Part model, mm, in its own coordinate system. Face numbers are marked on the shaded views. A direction names the side the tool comes from. Give positions to 0.01 mm unless a question says otherwise; leave off trailing zeros. Loops run counter-clockwise (first coordinate to the right, second up) from the corner with the lowest first, then second, coordinate; pieces in that order, holes last. Notation, with made-up numbers: M 79.25,70 L 83.25,70 A30 cw 83.25,105 Z; hole C -18,17.5 d4. An arc over 180 degrees is marked long. Answer in a Markdown table with one row per item.
from build123d import *

# Parameters (mm, degrees)
F0_W     = 40
F0_H     = 5
F1_DEPTH = 50
F0_W_2   = 30
F0_H_2   = 30
F2_DEPTH = 5


with BuildPart() as f1:
    # F0 (on Top) → F1 (new body)
    with BuildSketch(Plane.XY):
        Polygon((25, 10), (-25, 10), (-25, 0), (-15, 0), (15, 0), (25, 0), align=None)
        with Locations((0, 5)):
            Rectangle(F0_W, F0_H, mode=Mode.SUBTRACT)
    extrude(amount=F1_DEPTH)

    # F0 (on Top) → F2 (join)
    with BuildSketch(Plane.XY):
        with Locations((0, -15)):
            Rectangle(F0_W_2, F0_H_2)
        with Locations((0, 5)):
            Rectangle(F0_W, F0_H)
    extrude(amount=F2_DEPTH)


solid = f1.part
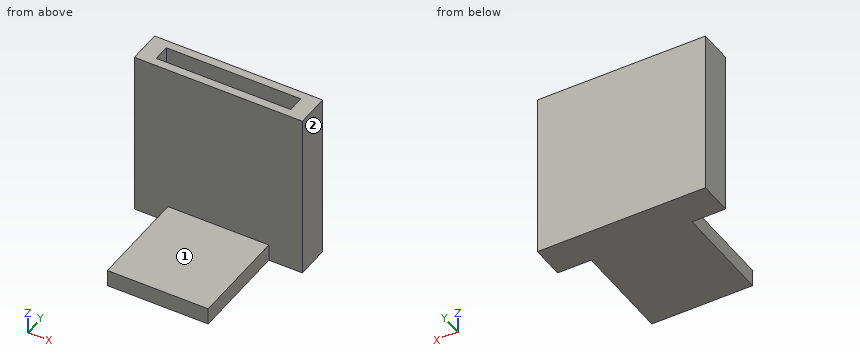
(1) Saw through at B-B (x = -16.5). Write the cut outline in (y, z), plus the area to 3 significant figures.
Recorded:
| item | result |
|---|---|
| outline | M 0,0 L 10,0 L 10,50 L 7.5,50 L 7.5,5 L 2.5,5 L 2.5,50 L 0,50 Z |
| area | 275 mm^2 |
(2) Saw through at C-C (y = 3.5). Write the cut outline in (x, z).
Recorded:
| item | result |
|---|---|
| outline | M -25,0 L 25,0 L 25,50 L 20,50 L 20,5 L -20,5 L -20,50 L -25,50 Z |
(3) Which spindle directions (+Z, -Z, +X, -X, +Y, -Y) get a long thin tool onto all of the face, cutting with end or side? Do the marked faces 1 and 2. Say none if no direction does.
Recorded:
| item | result |
|---|---|
| face 1 | +Z, +X, -X, -Y |
| face 2 | +Z, -Z, +X, +Y, -Y |
(4) Saw through at A-A (z = 8). Write the cut outline in (x, y), plus the area to 3 significant figures.
Recorded:
| item | result |
|---|---|
| outline | M -25,0 L 25,0 L 25,10 L -25,10 Z; hole M -20,2.5 L 20,2.5 L 20,7.5 L -20,7.5 Z |
| area | 300 mm^2 |
(5) Drill centre lines: line 1 along X through (y, z) = (7, 45); line 2 along Y through (x, z) = (-10, 11.5); line 3 along Z through (x, y) = (-1, -3). Where is each one in solid material? Low to high.
Recorded:
| item | result |
|---|---|
| line 1 | x = -25 to -20, 20 to 25 |
| line 2 | y = 0 to 2.5, 7.5 to 10 |
| line 3 | z = 0 to 5 |
(6) Pin check, flat tips, straight feed: pin 1 Ø2.5 at (y, z) = (-22, 3.5) entering from -X; pin 2 Ø1 at (x, z) = (15, 42.5) entering from -Y; pin 3 Ø4 at (x, y) = (-5, 5) entering from +Z. Stop position of each tip, or through.
Recorded:
| item | result |
|---|---|
| pin 1 | stops at x = -15 |
| pin 2 | stops at y = 0 |
| pin 3 | stops at z = 5 |
(7) Saw through at D-D (x = 1.5). Write the cut outline in (y, z), plus the area to 3 significant figures.
Recorded:
| item | result |
|---|---|
| outline | M -30,0 L 10,0 L 10,50 L 7.5,50 L 7.5,5 L 2.5,5 L 2.5,50 L 0,50 L 0,5 L -30,5 Z |
| area | 425 mm^2 |
